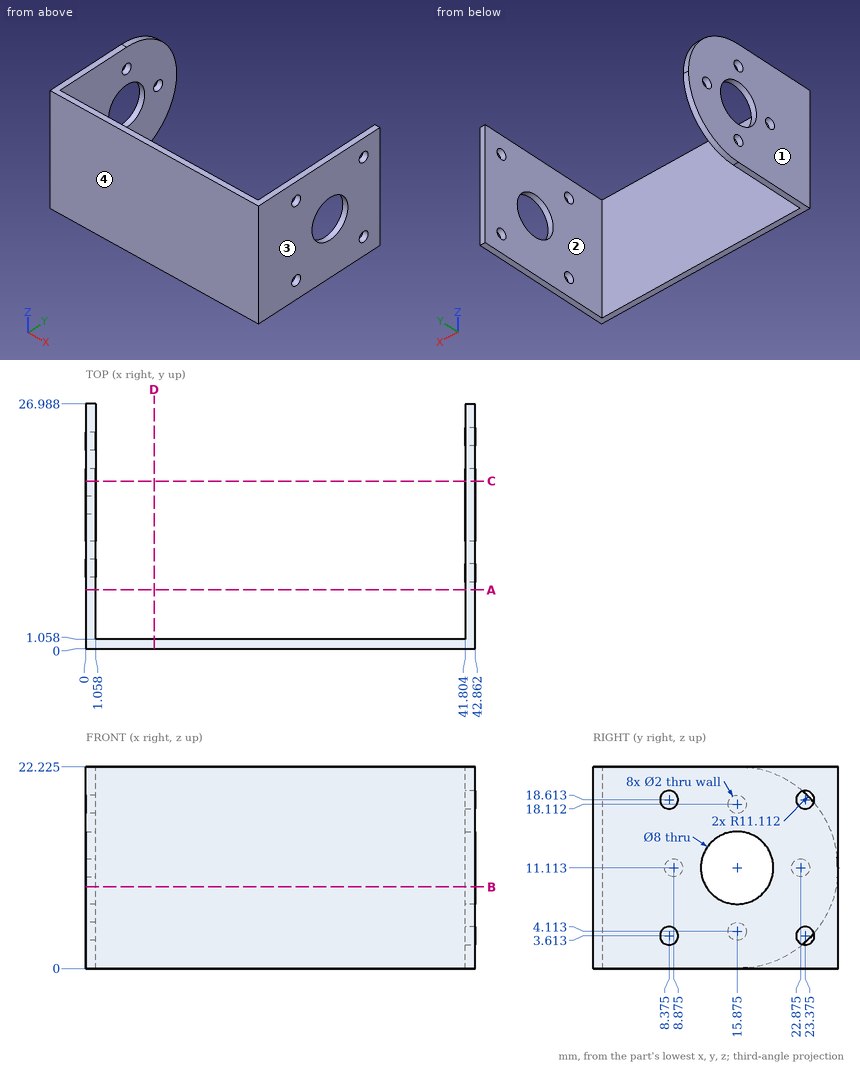
Can you work these out from the drawing? Everything is in mm from the part's minimum corner. Coordinates: 2 decimals unless noted, no trailing zeros. Loops run counter-clockwise (first coordinate to the right, second up) from the corner with the lowest first, then second, coordinate; pieces in that order, holes last.
1. Imagine slicing it at A-A, the plane y = 6.5. Please give me the cut outline in (x, z) (1 decimal).
2. Imagine slicing it at D-D, the plane x = 7.5. Please give me the cut outline in (y, z) (1 decimal).
3. Imagine slicing it at C-C, the plane y = 18.5. Please give me the cut outline in (x, z) (1 decimal).
4. I need wall thicknesses on L1, parallel to X at y = 2, z = 9.5 (1 decimal); L2, parallel to Y at x = 33, z = 15.5. Which ranges of each line are inside material? Lowest first, please.
5. Imagine slicing it at B-B, the plane z = 9. Please give me the cut outline in (x, y) (1 decimal).
6. If we mould it in two halves opening along X, with no side actions, what happens to the marked faces 1, 2, 3 and 4? For each: pulls with the +X half, pulls with the -X half, needs draft (parallel to the pull), parting line crosses it, or undercut.
7. For P1, Ø1.2, axis at y = 8.38, z = 18.61, coming from the +X side; P2, Ø6.5, axis at y = 15.88, z = 11.11, coming from the +X side; P3, Ø3, axis at x = 11.5, z = 9.5, coming from the +Y side, each with a flat end and sliding along its axis, tell me the tip position at first contact or that it passes through.
Taken from the geometry:
1. outline: (0, 0) - (1.1, 0) - (1.1, 22.2) - (0, 22.2) - close; (41.8, 0) - (42.9, 0) - (42.9, 22.2) - (41.8, 22.2) - close
2. outline: (0, 0) - (1.1, 0) - (1.1, 22.2) - (0, 22.2) - close
3. outline: (0, 0.3) - (1.1, 0.3) - (1.1, 8.1) - (0, 8.1) - close; (0, 14.1) - (1.1, 14.1) - (1.1, 21.9) - (0, 21.9) - close; (41.8, 0) - (42.9, 0) - (42.9, 8.1) - (41.8, 8.1) - close; (41.8, 14.1) - (42.9, 14.1) - (42.9, 22.2) - (41.8, 22.2) - close
4. L1: x = 0 to 1.1, 41.8 to 42.9
4. L2: y = 0 to 1.06
5. outline: (0, 0) - (42.9, 0) - (42.9, 12.5) - (41.8, 12.5) - (41.8, 1.1) - (1.1, 1.1) - (1.1, 12.5) - (0, 12.5) - close; (0, 19.3) - (1.1, 19.3) - (1.1, 26.8) - (0, 26.8) - close; (41.8, 19.3) - (42.9, 19.3) - (42.9, 27) - (41.8, 27) - close
6. face 1: pulls with the -X half
6. face 2: undercut
6. face 3: pulls with the +X half
6. face 4: needs draft
7. P1: stops at x = 1.06
7. P2: passes through
7. P3: stops at y = 1.06
